CAD build for the part. Positions are in the model's coordinates, mm. Face numbers are marked on the shaded views. A direction names the side the tool comes from. Give positions to 0.01 mm unless a question says otherwise; leave off trailing zeros. Loops run counter-clockwise (first coordinate to the right, second up) from the corner with the lowest first, then second, coordinate; pieces in that order, holes last. Notation, with made-up numbers: (-31, -33.75) - (12, -33.75) arc R32 cw to (12, 1.25) - close; hole circle Ø10 at (44.25, 77.25). An arc over 180 degrees is marked (long way). Return JSON: item names as keys, results as strings.
from build123d import *

# Parameters (mm, degrees)
F0_R      = 9
F1_DEPTH  = 24.5
F2_R      = 9
F3_DEPTH  = 14
F4_R      = 30
F5_DEPTH  = 6
F6_R      = 64.5
F8_DEPTH  = 30
F7_R      = 12
F7_R_2    = 6.35
F9_DEPTH  = 2
F10_DEPTH = 8


with BuildPart() as f1:
    # F0 (on Front) → F1 (new body, symmetric)
    with BuildSketch(Plane.XZ):
        with BuildLine():
            Line((-60, -70), (60, -70))
            ThreePointArc((60, -70), (67.0710678119, -67.0710678119), (70, -60))
            Line((70, -60), (70, 60))
            ThreePointArc((70, 60), (67.0710678119, 67.0710678119), (60, 70))
            Line((60, 70), (-60, 70))
            ThreePointArc((-60, 70), (-67.0710678119, 67.0710678119), (-70, 60))
            Line((-70, 60), (-70, -60))
            ThreePointArc((-70, -60), (-67.0710678119, -67.0710678119), (-60, -70))
        make_face()
        with Locations((-55, -55)):
            Circle(F0_R, mode=Mode.SUBTRACT)
        with Locations((55, -55)):
            Circle(F0_R, mode=Mode.SUBTRACT)
        with Locations((-55, 55)):
            Circle(F0_R, mode=Mode.SUBTRACT)
        with Locations((55, 55)):
            Circle(F0_R, mode=Mode.SUBTRACT)
    extrude(amount=F1_DEPTH, both=True)

    # F2 (on face) → F3 (cut)
    with BuildSketch(Plane.XZ.offset(24.5)):
        with BuildLine():
            Line((30, -50), (30, -70))
            Line((30, -70), (60, -70))
            ThreePointArc((60, -70), (67.0710678119, -67.0710678119), (70, -60))
            Line((70, -60), (70, -30))
            Line((70, -30), (50, -30))
            ThreePointArc((50, -30), (35.8578643763, -35.8578643763), (30, -50))
        make_face()
        with Locations((55, -55)):
            Circle(F2_R, mode=Mode.SUBTRACT)
        with BuildLine():
            Line((60, 70), (30, 70))
            Line((30, 70), (30, 50))
            ThreePointArc((30, 50), (35.8578643763, 35.8578643763), (50, 30))
            Line((50, 30), (70, 30))
            Line((70, 30), (70, 60))
            ThreePointArc((70, 60), (67.0710678119, 67.0710678119), (60, 70))
        make_face()
        with Locations((55, 55)):
            Circle(F2_R, mode=Mode.SUBTRACT)
        with BuildLine():
            Line((-70, 60), (-70, 30))
            Line((-70, 30), (-50, 30))
            ThreePointArc((-50, 30), (-35.8578643763, 35.8578643763), (-30, 50))
            Line((-30, 50), (-30, 70))
            Line((-30, 70), (-60, 70))
            ThreePointArc((-60, 70), (-67.0710678119, 67.0710678119), (-70, 60))
        make_face()
        with Locations((-55, 55)):
            Circle(F2_R, mode=Mode.SUBTRACT)
        with BuildLine():
            Line((-50, -30), (-70, -30))
            Line((-70, -30), (-70, -60))
            ThreePointArc((-70, -60), (-67.0710678119, -67.0710678119), (-60, -70))
            Line((-60, -70), (-30, -70))
            Line((-30, -70), (-30, -50))
            ThreePointArc((-30, -50), (-35.8578643763, -35.8578643763), (-50, -30))
        make_face()
        with Locations((-55, -55)):
            Circle(F2_R, mode=Mode.SUBTRACT)
    extrude(amount=-F3_DEPTH, mode=Mode.SUBTRACT)

    # F4 (on face) → F5 (join)
    with BuildSketch(Plane.XZ.offset(24.5)):
        Circle(F4_R)
    extrude(amount=F5_DEPTH)

    # F6 (on face) → F8 (cut)
    with BuildSketch(Plane(origin=(0, 24.5, 0), x_dir=(-1, 0, 0), z_dir=(0, 1, 0))):
        Circle(F6_R)
    extrude(amount=-F8_DEPTH, mode=Mode.SUBTRACT)

    # F7 (on face) → F9 (cut)
    with BuildSketch(Plane.YZ.offset(70)):
        with Locations((8.5, 7.547759451)):
            Circle(F7_R)
        with Locations((8.5, 7.547759451)):
            Circle(F7_R_2, mode=Mode.SUBTRACT)
    extrude(amount=-F9_DEPTH, mode=Mode.SUBTRACT)

    # F10 (cut): a face of the model
    f10_faces = [f1.faces().sort_by_distance(p)[0] for p in [
        (70, 8.5, 7.547759451),
    ]]
    extrude(f10_faces, amount=-F10_DEPTH, mode=Mode.SUBTRACT)


solid = f1.part
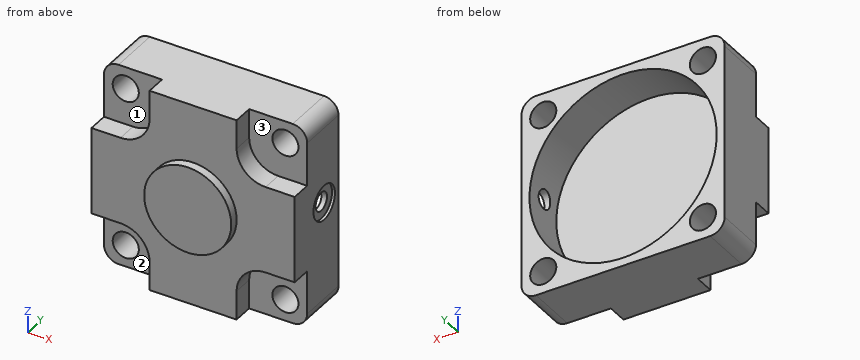
1. Cut at C-C, the plane z = -14. Write the cut outline in (x, y), plus the area to 3 significant figures.
Values follow:
{"outline": "(-70, -24.5) - (-26.53, -24.5) - (-26.53, -30.5) - (26.53, -30.5) - (26.53, -24.5) - (70, -24.5) - (70, 24.5) - (62.96, 24.5) - (62.96, -5.5) - (-62.96, -5.5) - (-62.96, 24.5) - (-70, 24.5) - close", "area": "3,400 mm²"}
2. Cut at A-A, the plane x = -55. Write the cut outline in (y, z), plus the area to 3 significant figures.
Values follow:
{"outline": "(-24.5, -30) - (-10.5, -30) - (-10.5, -46) - (24.5, -46) - (24.5, -33.69) - (-5.5, -33.69) - (-5.5, 33.69) - (24.5, 33.69) - (24.5, 46) - (-10.5, 46) - (-10.5, 30) - (-24.5, 30) - close; (-10.5, -70) - (24.5, -70) - (24.5, -64) - (-10.5, -64) - close; (-10.5, 64) - (24.5, 64) - (24.5, 70) - (-10.5, 70) - close", "area": "2,460 mm²"}
3. Cut at D-D, the plane y = 8.5. Write the cut outline in (x, z).
Values follow:
{"outline": "(-70, -60) arc R10 ccw to (-60, -70) - (60, -70) arc R10 ccw to (70, -60) - (70, -4.45) - (68, -4.45) - (68, 1.2) - (64.49, 1.2) arc R64.5 cw (long way) to (62.98, 13.9) - (68, 13.9) - (68, 19.55) - (70, 19.55) - (70, 60) arc R10 ccw to (60, 70) - (-60, 70) arc R10 ccw to (-70, 60) - close; hole circle Ø18 at (-55, -55); hole circle Ø18 at (-55, 55); hole circle Ø18 at (55, -55); hole circle Ø18 at (55, 55)"}
4. Cut at B-B, the plane y = -19. Write the cut outline in (x, z).
Values follow:
{"outline": "(-70, -30) - (-50, -30) arc R20 cw to (-30, -50) - (-30, -70) - (30, -70) - (30, -50) arc R20 cw to (50, -30) - (70, -30) - (70, 30) - (50, 30) arc R20 cw to (30, 50) - (30, 70) - (-30, 70) - (-30, 50) arc R20 cw to (-50, 30) - (-70, 30) - close"}
5. Drop flat-ended pins along their axis: P1, Ø11, axis at y = -16.5, z = -63, coming from the +X side; P2, Ø23.5, axis at x = -55, z = 55, coming from the -Y side; P3, Ø2, axis at x = 47.5, z = -20, coming from the -Y side. Give the stop position or say it passes through.
Values follow:
{"P1": "stops at x = 30", "P2": "stops at y = -10.5", "P3": "stops at y = -24.5"}
6. Which spindle directions (+Z, -Z, +X, -X, +Y, -Y) get a long thin tool onto all of the face, cutting with end or side? Do the marked faces 1, 2 and 3. Say none if no direction does.
Values follow:
{"face 1": "+Z, -X, -Y", "face 2": "-Z, -X, -Y", "face 3": "+Z, +X, -Y"}
7. Drill centre lines: probe 1 along Z at (x, y) = (0.5, 14.5); probe 2 along Z at (x, y) = (-55, 2.5); probe 3 along X at (y, z) = (13, 58). Where is each one in solid material? Low to high.
Values follow:
{"probe 1": "z = -70 to -64.5, 64.5 to 70", "probe 2": "z = -70 to -64, -46 to -33.69, 33.69 to 46, 64 to 70", "probe 3": "x = -70 to -63.49, -46.51 to -28.22, 28.22 to 46.51, 63.49 to 70"}
